Work out the finished part from the listing and answer in its coordinate system (mm). Coordinates: 2 decimals unless noted, no trailing zeros. Order: outer loops, then holes, each group sorted by start corner. A loop starts at its lowest first (then second) coordinate and runs counter-clockwise, first axis right, second up.
1. The part is cut by section D-D, the plane y = 19.5. Give the vertices of the cut face in (x, z).
2. Find the intervals of material crossed by probe 1 along Z at (x, y) = (-0.8, 19.5); probe 2 along Y at (x, z) = (1, 0); probe 3 along Z at (x, y) = (-0.35, -8), in increasing order.
3. The part is cut by section B-B, the plane y = -8. Give the vertices of the cut face in (x, z), then the cut area to 3 significant figures.
4. The part is cut by section A-A, the plane z = 0. Give the vertices of the cut face in (x, y), then the cut area to 3 significant figures.
5. The part is cut by section C-C, the plane x = 0.15. Give the vertices of the cut face in (y, z).
6. A flat-ended cylindrical pin translates along its axis: pin 1 Ø5 at (y, z) = (19.5, 13.5) entering from +X. Find the tip coordinate at first contact, or state that the pin passes through.
Autodesk Inventor part; units mm, degrees
ref_plane "YZ Plane" through (0, 0, 0) normal (1, 0, 0) x (0, 1, 0)
ref_plane "XZ Plane" through (0, 0, 0) normal (0, 1, 0) x (-1, 0, 0)
ref_plane "XY Plane" through (0, 0, 0) normal (0, 0, 1) x (1, 0, 0)
sketch "Skizze1" plane through (0, 0, 0) normal (1, 0, 0) x (0, 1, 0)
  line L0 (0, -30.1) -> (0, 30.1)
  line L1 (-41.3, 0) -> (41.3, 0)
  line L2 (-27.5, 21.5) -> (27.5, 21.5)
  line L3 (29.5, 19.5) -> (29.5, -19.5)
  line L4 (27.5, -21.5) -> (-27.5, -21.5)
  line L5 (-29.5, -19.5) -> (-29.5, 19.5)
  circle A0 centre (19.5, 13.5) radius 2.75
  circle A1 centre (19.5, -13.5) radius 2.75
  line L6 (27.5, 21.5) -> (29.5, 19.5)
  line L7 (29.5, -19.5) -> (27.5, -21.5)
  line L8 (-27.5, 21.5) -> (-29.5, 19.5)
  line L9 (-27.5, -21.5) -> (-29.5, -19.5)
  line L10 (8.6314, 16.6314) -> (6.3686, 14.3686) construction
  line L11 (7.5, 17.7627) -> (5.2373, 15.5)
  line L12 (7.5, 13.2373) -> (9.7627, 15.5)
  arc A2 (9.7627, 15.5) -> (7.5, 17.7627) centre (8.6314, 16.6314) ccw
  arc A3 (5.2373, 15.5) -> (7.5, 13.2373) centre (6.3686, 14.3686) ccw
  line L13 (-24.6314, 16.6314) -> (-22.3686, 14.3686) construction
  line L14 (-25.7627, 15.5) -> (-23.5, 13.2373)
  line L15 (-21.2373, 15.5) -> (-23.5, 17.7627)
  arc A4 (-23.5, 17.7627) -> (-25.7627, 15.5) centre (-24.6314, 16.6314) ccw
  arc A5 (-23.5, 13.2373) -> (-21.2373, 15.5) centre (-22.3686, 14.3686) ccw
  line L16 (8.6314, -16.6314) -> (6.3686, -14.3686) construction
  line L17 (9.7627, -15.5) -> (7.5, -13.2373)
  line L18 (5.2373, -15.5) -> (7.5, -17.7627)
  arc A6 (7.5, -17.7627) -> (9.7627, -15.5) centre (8.6314, -16.6314) ccw
  arc A7 (7.5, -13.2373) -> (5.2373, -15.5) centre (6.3686, -14.3686) ccw
  line L19 (-23.4997, -15.4997) -> (-23.5003, -15.5003) construction
  line L20 (-25.3683, -16.631) -> (-25.369, -16.6317)
  line L21 (-27.6317, -14.369) -> (-27.631, -14.3683)
  line L22 (-24.9849, -16.9849) -> (-22.0151, -14.0151) construction
  line L23 (-23.8536, -18.1163) -> (-20.8837, -15.1464)
  line L24 (-23.1464, -12.8837) -> (-26.1163, -15.8536)
  arc A8 (-26.1163, -15.8536) -> (-23.8536, -18.1163) centre (-24.9849, -16.9849) ccw
  arc A9 (-20.8837, -15.1464) -> (-23.1464, -12.8837) centre (-22.0151, -14.0151) ccw
  circle A10 centre (-8, 0) radius 12
  point P0 (0, 0)
  point P1 (-29.5, 21.5)
  point P2 (29.5, -21.5)
  point P3 (29.5, 21.5)
  point P4 (-29.5, -21.5)
  point P5 (7.5, 15.5)
  point P6 (-23.5, 15.5)
  point P7 (7.5, -15.5)
  point P8 (-23.5, -15.5)
  dimension "d0" = 59
  dimension "d1" = 43
  dimension "d2" = 5.5
  dimension "d3" = 10
  dimension "d4" = 8
  dimension "d14" = 2
  dimension "d15" = 2
  dimension "d16" = 2
  dimension "d17" = 2
  dimension "d18" = 2
  dimension "d19" = 2
  dimension "d20" = 2
  dimension "d21" = 2
  dimension "d22" = 3.2
  dimension "d23" = 3.2
  dimension "d24" = 3.2
  dimension "d26" = 6
  dimension "d27" = 31
  dimension "d28" = 31
  dimension "d31" = 2.1
  dimension "d32" = 3.2
  dimension "d35" = 24
  dimension "d36" = 15.5
extrude "Extrusion4" add sketch "Skizze1" along normal mid plane 3 contours L4 L9 L5 L1 A10 L0 | L0 A10 L1 L3 L7 L4 | L1 L5 L8 L2 L0 A10 | A10 L0 L2 L6 L3 L1
properties part number "Nema17_Montageplatte_Z-Achse" material "Aluminium 6061"
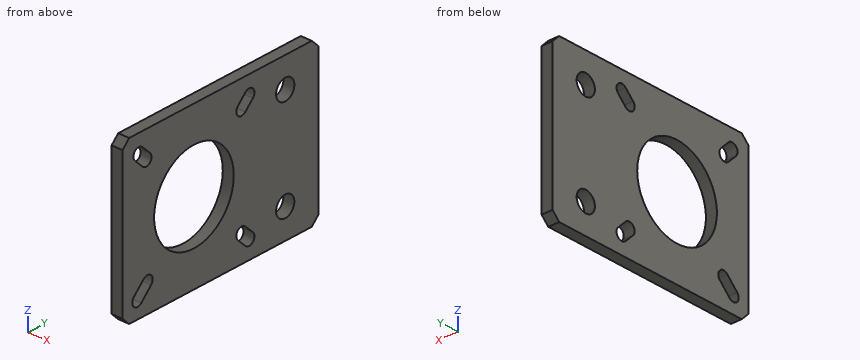
Geometry says:
1. outline: (-1.5, -21.5) - (1.5, -21.5) - (1.5, -16.25) - (-1.5, -16.25) - close; (-1.5, -10.75) - (1.5, -10.75) - (1.5, 10.75) - (-1.5, 10.75) - close; (-1.5, 16.25) - (1.5, 16.25) - (1.5, 21.5) - (-1.5, 21.5) - close
2. probe 1: z = -21.5 to -16.25, -10.75 to 10.75, 16.25 to 21.5
2. probe 2: y = -29.5 to -20, 4 to 29.5
2. probe 3: z = -21.5 to -12, 12 to 21.5
3. outline: (-1.5, -21.5) - (1.5, -21.5) - (1.5, -12) - (-1.5, -12) - close; (-1.5, 12) - (1.5, 12) - (1.5, 21.5) - (-1.5, 21.5) - close
3. area: 57.0 mm2
4. outline: (-1.5, -29.5) - (1.5, -29.5) - (1.5, -20) - (-1.5, -20) - close; (-1.5, 4) - (1.5, 4) - (1.5, 29.5) - (-1.5, 29.5) - close
4. area: 105 mm2
5. outline: (-29.5, -19.5) - (-27.5, -21.5) - (27.5, -21.5) - (29.5, -19.5) - (29.5, 19.5) - (27.5, 21.5) - (-27.5, 21.5) - (-29.5, 19.5) - close; hole (-26.12, -15.85) arc R1.6 ccw to (-23.85, -18.12) - (-20.88, -15.15) arc R1.6 ccw to (-23.15, -12.88) - close; hole (-25.76, 15.5) - (-23.5, 13.24) arc R1.6 ccw to (-21.24, 15.5) - (-23.5, 17.76) arc R1.6 ccw to start; hole circle Ø24 at (-8, 0); hole (5.24, -15.5) - (7.5, -17.76) arc R1.6 ccw to (9.76, -15.5) - (7.5, -13.24) arc R1.6 ccw to start; hole (5.24, 15.5) arc R1.6 ccw to (7.5, 13.24) - (9.76, 15.5) arc R1.6 ccw to (7.5, 17.76) - close; hole circle Ø5.5 at (19.5, -13.5); hole circle Ø5.5 at (19.5, 13.5)
6. pin 1: passes through
